Source: CAD feature listing. Evaluate the final solid. Frame: model axes, mm. Face numbers are marked on the shaded views. A direction names the side the tool comes from. Give positions to 0.01 mm unless a question says otherwise; leave off trailing zeros. Order: outer loops, then holes, each group sorted by start corner. A loop starts at its lowest first (then second) coordinate and runs counter-clockwise, first axis right, second up. Notation, with made-up numbers: M 30,43 L 62,43 A28 cw 62,67 Z; hole C 21,40.5 d9. An arc over 180 degrees is marked long. Return JSON: item names as keys, results as strings.
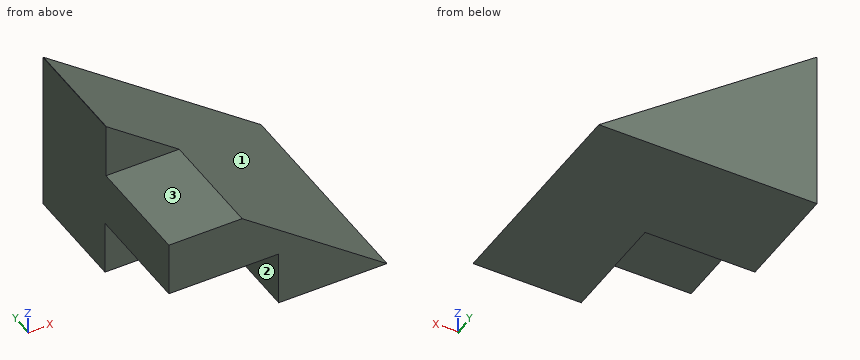
from build123d import *

# Parameters (mm, degrees)
F0_W     = 25.4
F0_H     = 6.35
F1_DEPTH = 38.1
F3_DEPTH = 25.4
F4_W     = 12.91742
F4_H     = 6.35
F5_DEPTH = 12.7
F7_DEPTH = 25.4


with BuildPart() as f1:
    # F0 (on Front) → F1 (new body)
    with BuildSketch(Plane.XZ):
        with Locations((12.7, 3.175)):
            Rectangle(F0_W, F0_H)
    extrude(amount=F1_DEPTH)

    # F2 (on Right) → F3 (join)
    with BuildSketch(Plane.YZ):
        Polygon((0, 6.330987), (0, 25.380987), (-12.7, 25.380987), (-12.7, 19.05), (-25.4, 19.05), (-25.4, 6.330987), (-12.7, 6.330987), align=None)
    extrude(amount=F3_DEPTH)

    # F4 (on Right) → F5 (cut)
    with BuildSketch(Plane.YZ):
        with Locations((-18.979252, 9.588845)):
            Rectangle(F4_W, F4_H)
    extrude(amount=F5_DEPTH, mode=Mode.SUBTRACT)

    # F6 (on Front) → F7 (intersect)
    with BuildSketch(Plane.XZ):
        Polygon((25.21595, 6.447089), (0, 25.42259), (0, 6.447089), align=None)
    extrude(amount=F7_DEPTH, mode=Mode.INTERSECT)


solid = f1.part
1. Section query A-A (x = 3). Return loops of the section in (y, z), then the cut area to 3 significant figures.
Evaluation:
{"outline": "M -25.4,12.76 L -12.52,12.76 L -12.52,6.45 L 0,6.45 L 0,23.17 L -12.7,23.17 L -12.7,19.05 L -25.4,19.05 Z", "area": "291 mm^2"}
2. Section query D-D (x = 6.25). Return loops of the section in (y, z).
Evaluation:
{"outline": "M -25.4,12.76 L -12.52,12.76 L -12.52,6.45 L 0,6.45 L 0,20.72 L -12.7,20.72 L -12.7,19.05 L -25.4,19.05 Z"}
3. Set-up query: the marked faces 1, 2 and 3. Return all of +Z, -Z, +X, -X, +Y, -Y with unobstructed straight access to the full face (end or side cutting, diameter ignored); none if empty.
Evaluation:
{"face 1": "+Z, +X, +Y, -Y", "face 2": "-Z, -X, -Y", "face 3": "+Z, +X, -X, -Y"}
4. Ray query, probe 1 along Y at (x, z) = (4.5, 9.5); probe 2 along Z at (x, y) = (4.5, -20); probe 3 along Y at (x, z) = (1, 19.75). Return the intervals inside material, ascending.
Evaluation:
{"probe 1": "y = -12.52 to 0", "probe 2": "z = 12.76 to 19.05", "probe 3": "y = -12.7 to 0"}
5. First-contact query: pin 1 (5 mm diameter, centred on y = -18, z = 8, fed in from -X); pin 2 (4 mm diameter, centred on y = -18.5, z = 14, fed in from -X); pin 3 (5 mm diameter, centred on x = 4, z = 23.5, fed in from -Y); pin 4 (4 mm diameter, centred on x = 2.5, y = -21, fed in from +Z). Flat tips, straight axial feed; report the tip coordinate or a pass-through.
Evaluation:
{"pin 1": "stops at x = 12.7", "pin 2": "stops at x = 0", "pin 3": "stops at y = -12.7", "pin 4": "stops at z = 19.05"}
6. Section query B-B (y = -21.75). Return loops of the section in (x, z).
Evaluation:
{"outline": "M 0,12.76 L 12.7,12.76 L 12.7,6.45 L 25.22,6.45 L 8.47,19.05 L 0,19.05 Z"}
7. Section query C-C (z = 9.5). Return loops of the section in (x, y).
Evaluation:
{"outline": "M 0,-12.52 L 12.7,-12.52 L 12.7,-25.4 L 21.16,-25.4 L 21.16,0 L 0,0 Z"}
